For this review, take the finished solid that the model builds, in its own axes (mm). A direction names the side the tool comes from. Coordinates: 2 decimals unless noted, no trailing zeros. Order: outer loops, then holes, each group sorted by start corner. A loop starts at its lowest first (then second) coordinate and runs counter-clockwise, first axis right, second up. Notation, with made-up numbers: (-8, 34.25) -> (44, 34.25) arc R8 ccw to (44, 46.25) -> close; hole circle Ø4 at (82.25, -3). An arc over 180 degrees is marked (long way). Write item = value, one per line. Start each with the question number.
1) Consider section A-A on x = 8. Give the boundary of the cut face in (y, z), and give its area (3 significant figures).
2) Wall thickness on probe 1 along X at (y, z) = (19, 1); probe 2 along Y at (x, z) = (15.5, -2.5); probe 3 along Z at (x, y) = (25.5, 15.5): over which ranges is each line inside the solid? List them lowest first. Write a range as [from, to].
3) Consider section B-B on z = -19.05. Give the boundary of the cut face in (x, y).
4) Insertion check: pin 1 Ø5 at (x, z) = (24.5, -6) entering from +Y; pin 2 Ø4 at (x, y) = (5.5, 13) entering from -Z. Each pin has a flat end and moves straight along its axis. Give the tip position at first contact, or say it passes through.
5) Consider section D-D on x = 14. Give the boundary of the cut face in (y, z).
6) Machinability: for faces 4 (the face through (16, 0, -16)), 5 (the face through (0, 6, 2)), which of the approach directions +Z, -Z, +X, -X, +Y, -Y give a long, thin tool a straight path to every point of the face, cutting with its end or side? Answer none if there is none.
7) Consider section C-C on y = 19.05. Give the boundary of the cut face in (x, z).
8) Draft analysis for pull direction Z (two halves, no side actions). For faces 1 (the face through (6.89, -3.22, -18.04)), 2 (the face through (16, 13, 6.35)), 3 (the face through (16, 16, 0)), state which applies: +Z half, -Z half, draft (parallel to the pull), parting line (faces both ways), or undercut.
from build123d import *

# Parameters (mm, degrees)
BOSS_EXTRUDE1_DEPTH = 31.75
FILLET1_R           = 6
SKETCH2_R           = 1.5
CUT_EXTRUDE1_DEPTH  = 39.1
SKETCH3_R           = 1.5
CUT_EXTRUDE2_DEPTH  = 39.1
FILLET2_R           = 6


with BuildPart() as part:
    # Sketch1 → Boss-Extrude1 (new body)
    with BuildSketch(Plane(origin=(0, 0, 0), x_dir=(0, 0, -1), z_dir=(1, 0, 0))):
        Polygon((-6.35, 31.75), (-6.35, -6.35), (31.75, -6.35), (31.75, 0), (0, 0), (0, 31.75), align=None)
    extrude(amount=BOSS_EXTRUDE1_DEPTH)

    # Fillet1
    fillet1_edges = [part.edges().sort_by_distance(p)[0] for p in [
        (15.875, -6.35, -31.75),
        (15.875, 31.75, 6.35),
    ]]
    fillet(fillet1_edges, radius=FILLET1_R)

    # Sketch2 → Cut-Extrude1 (cut, through all)
    with BuildSketch(Plane.XY.offset(6.35)):
        with Locations((8, 19.05)):
            Circle(SKETCH2_R)
        with Locations((23.75, 19.05)):
            Circle(SKETCH2_R)
    extrude(amount=-CUT_EXTRUDE1_DEPTH, mode=Mode.SUBTRACT)

    # Sketch3 → Cut-Extrude2 (cut, through all)
    with BuildSketch(Plane.XZ.offset(6.35)):
        with Locations((8, -19.05)):
            Circle(SKETCH3_R)
        with Locations((23.75, -19.05)):
            Circle(SKETCH3_R)
    extrude(amount=-CUT_EXTRUDE2_DEPTH, mode=Mode.SUBTRACT)

    # Fillet2
    fillet2_edges = [part.edges().sort_by_distance(p)[0] for p in [
        (15.875, -6.35, 6.35),
    ]]
    fillet(fillet2_edges, radius=FILLET2_R)


solid = part.part
Answer sheet:
q1.outline = (-6.35, -25.75) arc R6 ccw to (-0.35, -31.75) -> (0, -31.75) -> (0, -20.55) -> (-6.35, -20.55) -> close; (-6.35, -17.55) -> (0, -17.55) -> (0, 0) -> (17.55, 0) -> (17.55, 6.35) -> (-0.35, 6.35) arc R6 ccw to (-6.35, 0.35) -> close; (20.55, 0) -> (31.75, 0) -> (31.75, 0.35) arc R6 ccw to (25.75, 6.35) -> (20.55, 6.35) -> close
q1.area = 382 mm2
q2.probe_1 = [0, 6.5], [9.5, 22.25], [25.25, 31.75]
q2.probe_2 = [-6.35, 0]
q2.probe_3 = [0, 6.35]
q3.outline = (0, -6.35) -> (6.5, -6.35) -> (6.5, 0) -> (0, 0) -> close; (9.5, -6.35) -> (22.25, -6.35) -> (22.25, 0) -> (9.5, 0) -> close; (25.25, -6.35) -> (31.75, -6.35) -> (31.75, 0) -> (25.25, 0) -> close
q4.pin_1 = 0
q4.pin_2 = 0
q5.outline = (-6.35, -25.75) arc R6 ccw to (-0.35, -31.75) -> (0, -31.75) -> (0, 0) -> (31.75, 0) -> (31.75, 0.35) arc R6 ccw to (25.75, 6.35) -> (-0.35, 6.35) arc R6 ccw to (-6.35, 0.35) -> close
q6.face_4 = -Z, +X, -X, +Y
q6.face_5 = +Z, -Z, -X, +Y, -Y
q7.outline = (0, 0) -> (6.5, 0) -> (6.5, 6.35) -> (0, 6.35) -> close; (9.5, 0) -> (22.25, 0) -> (22.25, 6.35) -> (9.5, 6.35) -> close; (25.25, 0) -> (31.75, 0) -> (31.75, 6.35) -> (25.25, 6.35) -> close
q8.face_1 = undercut
q8.face_2 = +Z half
q8.face_3 = -Z half
